Source: CAD feature listing. Evaluate the final solid. Frame: model axes, mm. A direction names the side the tool comes from. Round coordinates to 2 decimals unless told otherwise and drop trailing zeros. Order: outer loops, then holes, each group sorted by start corner. A loop starts at its lowest first (then second) coordinate and runs counter-clockwise, first axis right, second up.
Autodesk Inventor part; units mm, degrees
ref_plane "Work Plane2" through (2.032, 0, 0) normal (0, 1, 0) x (1, 0, 0)
ref_plane "YZ Plane" through (0, 0, 0) normal (1, 0, 0) x (0, 1, 0)
ref_plane "XZ Plane" through (0, 0, 0) normal (0, 1, 0) x (-1, 0, 0)
sketch "Sketch1" plane through (0, 0, 0) normal (0, 0, 1) x (1, 0, 0)
  line L0 (2.6924, 0) -> (7.9375, 0)
  line L1 (7.9375, 0) -> (7.9375, 1.7526)
  line L2 (7.9375, 1.7526) -> (2.1082, 1.7526)
  line L3 (0.5596, 3.0988) -> (0, 3.0988)
  line L4 (-1.5875, 0) -> (9.525, 0)
  line L5 (0, -0.6198) -> (0, 3.7186)
  line L6 (0, 2.2098) -> (2.0648, 1.1803)
  line L7 (2.0648, 1.1803) -> (2.6924, 0)
  line L8 (2.1082, 1.7526) -> (0.5596, 3.0988)
  line L9 (0, 3.0988) -> (0, 2.2098)
  dimension "d2" = 3.5052
  dimension "d3" = 6.1976
  dimension "d4" = 2.6924
  dimension "d5" = 4.4196
  dimension "d6" = 26.5
  dimension "d7" = 62
  dimension "d13" = 41
  dimension "d14" = 2.1082
  dimension "d15" = 7.9375
revolve "Body" add sketch "Sketch1" angle 360 about axis through (2.6924, 0, 0) along (1, 0, 0) contours L7 L6 L5 L3 L8 L2 L1 L0
sketch "Sketch2" plane through (0, 0, 0) normal (-1, 0, 0) x (0, 0, 1)
  line L0 (0, -4.3383) -> (0, 4.3383)
  line L1 (-4.3383, 0) -> (4.3383, 0)
  line L2 (0, 2.2098) -> (0, 0) construction
  line L3 (0, 0) -> (2.2098, 0) construction
  arc A0 (0.7366, 0) -> (0, 0.7366) centre (0, 0) ccw
  line L4 (0, 0) -> (0.7947, 0.7947) construction
  arc A1 (1.1049, 0) -> (0, 1.1049) centre (0, 0) ccw construction
  line L5 (0.3683, 2.1789) -> (0.3131, 1.0596)
  line L6 (2.1789, 0.3683) -> (1.0596, 0.3131)
  arc A2 (0.3131, 1.0596) -> (1.0596, 0.3131) centre (1.0245, 1.0245) ccw
  arc A3 (2.2098, 0) -> (2.1789, 0.3683) centre (0, 0) ccw
  arc A4 (0.3683, 2.1789) -> (0, 2.2098) centre (0, 0) ccw
  arc A5 (2.1789, 0.3683) -> (0.3683, 2.1789) centre (0, 0) ccw
  line L7 (0.3683, -2.1789) -> (0.3131, -1.0596)
  line L8 (2.1789, -0.3683) -> (1.0596, -0.3131)
  arc A6 (1.0596, -0.3131) -> (0.3131, -1.0596) centre (1.0245, -1.0245) ccw
  arc A7 (2.1789, -0.3683) -> (2.2098, 0) centre (0, 0) ccw
  arc A8 (0, -2.2098) -> (0.3683, -2.1789) centre (0, 0) ccw
  arc A9 (0.3683, -2.1789) -> (2.1789, -0.3683) centre (0, 0) ccw
  line L9 (-0.3683, 2.1789) -> (-0.3131, 1.0596)
  line L10 (-2.1789, 0.3683) -> (-1.0596, 0.3131)
  arc A10 (-1.0596, 0.3131) -> (-0.3131, 1.0596) centre (-1.0245, 1.0245) ccw
  arc A11 (-2.1789, 0.3683) -> (-2.2098, 0) centre (0, 0) ccw
  arc A12 (0, 2.2098) -> (-0.3683, 2.1789) centre (0, 0) ccw
  arc A13 (-0.3683, 2.1789) -> (-2.1789, 0.3683) centre (0, 0) ccw
  arc A14 (-2.1789, -0.3683) -> (-0.3683, -2.1789) centre (0, 0) ccw
  arc A15 (-0.3683, -2.1789) -> (0, -2.2098) centre (0, 0) ccw
  arc A16 (-2.2098, 0) -> (-2.1789, -0.3683) centre (0, 0) ccw
  line L11 (-2.1789, -0.3683) -> (-1.0596, -0.3131)
  arc A17 (-0.3131, -1.0596) -> (-1.0596, -0.3131) centre (-1.0245, -1.0245) ccw
  line L12 (-0.3683, -2.1789) -> (-0.3131, -1.0596)
  dimension "d18" = 45
  dimension "d19" = 1.4732
  dimension "d20" = 2.2098
  dimension "d21" = 4.4196
  dimension "d22" = 0.3683
extrude "Slot" add sketch "Sketch2" against normal up to next contours A2 L5 A5 L6 | L9 A10 L10 A13 | L7 A6 L8 A9 | A14 L11 A17 L12
fillet "Fillet1" radius 0.1473 4 edges at (0, 2.2098, 0) (0, 0, 2.2098) (0, -2.2098, 0) (0, 0, -2.2098)
thread "Thread"
chamfer "Chamfer1" distance 0.5953 distance2 0.5953 1 edges at (7.9375, -1.7526, 0) measured on face at (7.9375, -0.6726, -0.7284)
ref_plane "Work Plane2" through (2.032, 0, 0) normal (0, 1, 0) x (1, 0, 0)
equation "\"d2\" = GD"
equation "\"d3\" = KOD"
equation "\"d4\" = INTI"
equation "\"d5\" = SDM"
equation "\"d13\" = 0.5 * SEWI"
equation "\"d14\" = KOH"
equation "\"d15\" = NLG"
equation "\"d19\" = 0.333333 * SDM"
equation "\"d20\" = 0.5 * SDM"
equation "\"d21\" = SDM"
equation "\"d22\" = 0.5 * SBR"
equation "\"d45\" = INTI"
equation "\"d25\" = 0.2 * SBR"
equation "\"d9\" = GEL"
equation "\"d11\" = -0.5 * SPD + 0.5 * GD"
equation "\"d12\" = GUL"
equation "\"GD\" = NND"
equation "\"NLG\" = 7.9375"
equation "\"GEL\" = 3.84492"
equation "\"KOD\" = 6.1976"
equation "\"KOH\" = 2.1082"
equation "\"SDM\" = 4.4196"
equation "\"INTI\" = 2.6924"
equation "\"SBR\" = 0.7366"
equation "\"GUL\" = 0.75 * GAL"
equation "\"SPD\" = 2.31458"
equation "\"SEWI\" = 82deg"
equation "\"d0\" = NLG"
equation "\"d1\" = KOH"
equation "\"d17\" = SDM"
equation "\"TOA\" = 30deg"
equation "\"THREADDIA\" = 3.5052"
equation "\"BDM\" = NND"
equation "\"NND\" = 3.5052"
equation "\"GAL\" = 0.79375"
equation "\"GD1\" = SPD"
properties part number "ANSI B18.6.3 - 6-32 x 5/16, CRFCHMSTII(5)" material "Steel, Mild"
1. Section A-A on x = 1.25. Return loops of the section in (y, z).
2. Pull-direction query (Y, two-part tool) for faces 3 (the face through (4.69, 1.67, -0.53)), 4 (the face through (0.8, -1.4, 0.33)), 5 (the face through (7.938, 0, 0)); classes: released by +Y, released by -Y, zero draft, split by the parting line, or undercut.
3. First-contact query: pin 1 (2 mm diameter, centred on x = 3.5, z = -2, fed in from -Y); pin 2 (1.5 mm diameter, centred on x = 6.5, z = -1, fed in from -Y); pin 3 (1.5 mm diameter, centred on y = 1, z = -2, fed in from +X). Flat tips, straight axial feed; report the tip coordinate or a pass-through.
4. Access query for faces 1 (the face through (0, 1, -1)), 2 (the face through (1.06, -0.01, 1.68)). Directions: +Z, -Z, +X, -X, +Y, -Y. A direction counts if a zero-diameter tool reaches every point of the face in a straight line with its end or side. Return the directions, or none.
5. Section B-B on x = 4.25. Return loops of the section in (y, z).
6. Line query: line 1 along Y through (x, z) = (2, -0.25); line 2 along Y through (x, z) = (1, 1.5); line 3 along X through (y, z) = (0.25, -0.75). Output: solid intervals per line, ascending.
Result:
1. outline: circle Ø5 at (0, 0); hole (-1.55, -0.34) - (-1.06, -0.31) arc R0.71 cw to (-0.31, -1.06) - (-0.34, -1.55) arc R1.59 ccw to (0.34, -1.55) - (0.31, -1.06) arc R0.71 cw to (1.06, -0.31) - (1.55, -0.34) arc R1.59 ccw to (1.55, 0.34) - (1.06, 0.31) arc R0.71 cw to (0.31, 1.06) - (0.34, 1.55) arc R1.59 ccw to (-0.34, 1.55) - (-0.31, 1.06) arc R0.71 cw to (-1.06, 0.31) - (-1.55, 0.34) arc R1.59 ccw to start
2. face 3: split by the parting line
2. face 4: undercut
2. face 5: zero draft
3. pin 1: stops at y = -1.44
3. pin 2: stops at y = -1.73
3. pin 3: stops at x = 7.61
4. face 1: +Z, -Z, -X, +Y, -Y
4. face 2: -X
5. outline: circle Ø3.51 at (0, 0)
6. line 1: y = -1.83 to -1.19, 1.19 to 1.83
6. line 2: y = -2.26 to -0.33, 0.33 to 2.26
6. line 3: x = 2.27 to 7.94
